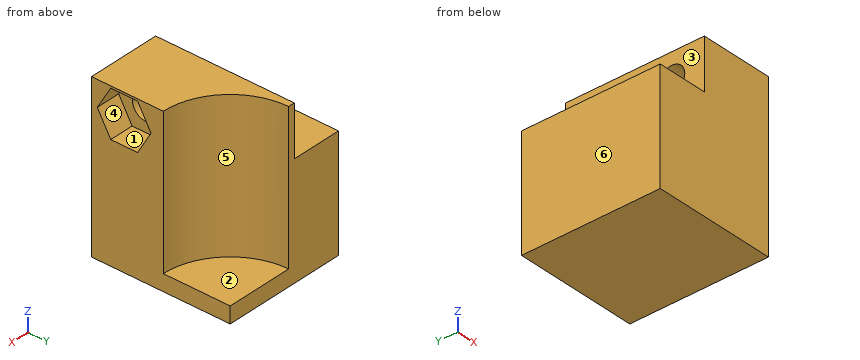
from build123d import *

# Parameters (mm, degrees)
CROQUIS1_W              = 15.2
CROQUIS1_H              = 17
SALIENTE_EXTRUIR1_DEPTH = 2
SALIENTE_EXTRUIR2_DEPTH = 11.8
SALIENTE_EXTRUIR3_DEPTH = 6.2
CORTAR_EXTRUIR1_REACH   = 11
CROQUIS4_R              = 1.6
CORTAR_EXTRUIR2_DEPTH   = 3


with BuildPart() as part:
    # Croquis1 → Saliente-Extruir1 (new body)
    with BuildSketch(Plane.XY):
        with Locations((7.6, 8.5)):
            Rectangle(CROQUIS1_W, CROQUIS1_H)
    extrude(amount=SALIENTE_EXTRUIR1_DEPTH)

    # Croquis2 → Saliente-Extruir2 (add)
    with BuildSketch(Plane.XY.offset(2)):
        with BuildLine():
            Line((0, 17), (0, 0))
            Line((0, 0), (15.2, 0))
            Line((15.2, 0), (15.2, 8.8))
            ThreePointArc((15.2, 8.8), (9.401724394, 11.201724394), (7, 17))
            Line((7, 17), (0, 17))
        make_face()
    extrude(amount=SALIENTE_EXTRUIR2_DEPTH)

    # Croquis3 → Saliente-Extruir3 (add)
    with BuildSketch(Plane.XY.offset(13.8)):
        with BuildLine():
            Line((6.2, 17), (6.2, 0))
            Line((6.2, 0), (15.2, 0))
            Line((15.2, 0), (15.2, 8.8))
            ThreePointArc((15.2, 8.8), (9.401724394, 11.201724394), (7, 17))
            Line((7, 17), (6.2, 17))
        make_face()
    extrude(amount=SALIENTE_EXTRUIR3_DEPTH)

    # Croquis4 → Cortar-Extruir1 (cut, up to next)
    with BuildSketch(Plane.ZY.offset(-6.2), mode=Mode.PRIVATE) as cortar_extruir1_sk1:
        with Locations((16.9, 4)):
            Circle(CROQUIS4_R)
    cortar_extruir1_tool1 = extrude(cortar_extruir1_sk1.sketch, amount=-CORTAR_EXTRUIR1_REACH, mode=Mode.PRIVATE) & part.part
    add(cortar_extruir1_tool1.solids().sort_by_distance((6.2, 4, 16.9))[0], mode=Mode.SUBTRACT)

    # Croquis5 → Cortar-Extruir2 (cut)
    with BuildSketch(Plane(origin=(15.2, 0, 0), x_dir=(0, 0, -1), z_dir=(1, 0, 0))):
        Polygon((-16.9, 0.709103466), (-14.05, 2.354551733), (-14.05, 5.645448267), (-16.9, 7.290896534), (-19.75, 5.645448267), (-19.75, 2.354551733), align=None)
    extrude(amount=-CORTAR_EXTRUIR2_DEPTH, mode=Mode.SUBTRACT)


solid = part.part
Verification items for the finished model (mm, model axes). Face numbers are marked on the shaded views. A direction names the side the tool comes from. Give positions to 0.01 mm unless a question says otherwise; leave off trailing zeros. Write each loop counter-clockwise with the first axis right and the second up, starting at its lowest first coordinate (ties: lowest second). Pieces come first, ordered by that corner, then holes. Notation, with made-up numbers: (55.5, 27.25) - (66.5, 27.25) arc R26 cw to (66.5, 66.25) - close; hole circle Ø2 at (-30, 87). An arc over 180 degrees is marked (long way). Answer as CSV lines item,"result". Start each with the question number.
1. Sectioned sample at B-B (z = 16). Record the boundary of the cut face in (x, y), then the cut area to 3 significant figures.
2. Sectioned sample at C-C (x = 13.25). Record the boundary of the cut face in (y, z).
3. Sectioned sample at A-A (y = 4). Record the boundary of the cut face in (x, z).
4. Set-up check for the marked faces 1, 2 and 3: record each of +Z, -Z, +X, -X, +Y, -Y from which the full face is reachable in a straight line by a thin tool's end or side.
5. Sectioned sample at D-D (z = 3.75). Record the boundary of the cut face in (x, y), then the cut area to 3 significant figures.
6. Depth check by flat-ended pin: pin 1 (5 mm diameter, centred on y = 4, z = 16.9, fed in from +X); pin 2 (1.9 mm diameter, centred on y = 7.5, z = 15.5, fed in from -X); pin 3 (7 mm diameter, centred on x = 2, y = 6.5, fed in from +Z). Enter the tip coordinate at first touch or a pass-through.
7. Thickness scan on line 1 (X direction, y = 5.75, z = 15.5); line 2 (Z direction, x = 12.75, y = 11); line 3 (Y direction, x = 9.55, z = 16.9). Record the ranges inside material, lowest first.
8. Draft check along Y on the marked faces 4, 5 and 6. Enter one of: pulls with the +Y half, pulls with the -Y half, needs draft (parallel to the pull), parting line crosses it, or undercut.
Derived:
1,outline,"(6.2, 0) - (15.2, 0) - (15.2, 1.23) - (12.2, 1.23) - (12.2, 2.68) - (6.2, 2.68) - close; (6.2, 5.32) - (12.2, 5.32) - (12.2, 6.77) - (15.2, 6.77) - (15.2, 8.8) arc R8.2 cw to (7, 17) - (6.2, 17) - close"
1,area,"67.7 mm²"
2,outline,"(0, 0) - (17, 0) - (17, 2) - (9.04, 2) - (9.04, 20) - (0, 20) - close; hole (0.71, 16.9) - (2.35, 14.05) - (5.65, 14.05) - (7.29, 16.9) - (5.65, 19.75) - (2.35, 19.75) - close"
3,outline,"(0, 0) - (15.2, 0) - (15.2, 14.05) - (12.2, 14.05) - (12.2, 15.3) - (6.2, 15.3) - (6.2, 13.8) - (0, 13.8) - close; (6.2, 18.5) - (12.2, 18.5) - (12.2, 19.75) - (15.2, 19.75) - (15.2, 20) - (6.2, 20) - close"
4,face 1,"+X"
4,face 2,"+Z, +X, +Y"
4,face 3,"+Z, -X, +Y, -Y"
5,outline,"(0, 0) - (15.2, 0) - (15.2, 8.8) arc R8.2 cw to (7, 17) - (0, 17) - close"
5,area,"206 mm²"
6,pin 1,"x = 12.2"
6,pin 2,"x = 6.2"
6,pin 3,"z = 13.8"
7,line 1,"6.2 to 12.2"
7,line 2,"0 to 2"
7,line 3,"0 to 2.4, 5.6 to 11.06"
8,face 4,"undercut"
8,face 5,"pulls with the +Y half"
8,face 6,"needs draft"
